from build123d import *

# Parameters (mm, degrees)
F0_W     = 152.4
F0_H     = 107.95
F1_DEPTH = 25.4
F2_SIZE2 = 50.8
F2_SIZE  = 25.4


with BuildPart() as f1:
    # F0 (on Top) → F1 (new body)
    with BuildSketch(Plane.XY):
        Rectangle(F0_W, F0_H)
    extrude(amount=F1_DEPTH)

    # F2
    f2_edges = [f1.edges().sort_by_distance(p)[0] for p in [
        (-76.2, 53.975, 12.7),
        (76.2, 53.975, 12.7),
    ]]
    chamfer(f2_edges, length=F2_SIZE, length2=F2_SIZE2)


solid = f1.part
Model file for the job. Use its own axes, mm. Round coordinates to 2 decimals unless told otherwise and drop trailing zeros. Order: outer loops, then holes, each group sorted by start corner. A loop starts at its lowest first (then second) coordinate and runs counter-clockwise, first axis right, second up.
(1) Drill centre lines: line 1 (Y direction, x = 31, z = 11.25) (3 decimals); line 2 (Y direction, x = 45.5, z = 11.5) (3 decimals); line 3 (X direction, y = 45, z = 22.75). Where is each one in solid material? Low to high.
(2) Band-saw the part on A-A (z = 11.25). List the corners of the cut face in (x, y) (3 decimals), then the cut area to 3 significant figures.
(3) Band-saw the part on C-C (x = 32.5). List the corners of the cut face in (y, z) (3 decimals), then the cut area to 3 significant figures.
(4) Band-saw the part on B-B (x = -56). List the corners of the cut face in (y, z) (3 decimals).
Verdict:
1. line 1: y = -53.975 to 51.175
1. line 2: y = -53.975 to 43.925
1. line 3: x = -43.35 to 43.35
2. outline: (-76.2, -53.975) - (76.2, -53.975) - (76.2, 28.575) - (25.4, 53.975) - (-25.4, 53.975) - (-76.2, 28.575) - close
2. area: 15,200 mm2
3. outline: (-53.975, 0) - (50.425, 0) - (50.425, 25.4) - (-53.975, 25.4) - close
3. area: 2,650 mm2
4. outline: (-53.975, 0) - (38.675, 0) - (38.675, 25.4) - (-53.975, 25.4) - close
